For this review, take the finished solid that the model builds, in its own axes (mm). Coordinates: 2 decimals unless noted, no trailing zeros. Order: outer loops, then holes, each group sorted by start corner. A loop starts at its lowest first (then second) coordinate and runs counter-clockwise, first axis right, second up. Notation, with made-up numbers: (-30.75, 9.25) -> (0.25, 9.25) arc R13 ccw to (0.25, 21.25) -> close; hole circle Ø5 at (-30.5, 4). An arc over 180 degrees is marked (long way). Return JSON: item names as keys, results as strings. Group by question number.
Item 1: Take a section at C-C (x = -7). Write out the cut boundary in (y, z) (3 decimals).
Item 2: Insertion check: pin 1 (1.5 mm diameter, centred on x = -26, y = 1, fed in from +Z). The pin has a flat end and moves straight along its axis. Give the tip position at first contact, or say it passes through.
Item 3: Take a section at D-D (z = 1). Write out the cut boundary in (x, y) (3 decimals), then the cut area to 3 significant figures.
Item 4: For line 1 along Z through (x, y) = (0, 0.7) (3 decimals); line 2 along X through (y, z) = (2.35, 15); line 3 along Z through (x, y) = (9, 1.65), list the stretches that pass through material, from the lowest coordinate up.
Item 5: Take a section at B-B (y = 2.6). Write out the cut boundary in (x, z) (3 decimals), then the cut area to 3 significant figures.
Item 6: Take a section at A-A (x = 0). Write out the cut boundary in (y, z) (3 decimals), then the cut area to 3 significant figures.
```python
from build123d import *

# Parameters (mm, degrees)
SKETCH1_W                = 25.4
SKETCH1_H                = 50.8
BOSS_EXTRUDE1_DEPTH      = 3.175
M5_CLEARANCE_HOLE1_D     = 5.5
M5_CLEARANCE_HOLE1_DEPTH = 12.7
M5_CLEARANCE_HOLE1_TIP   = 1.652366702
FILLET1_R                = 12.7
FILLET2_R                = 3.175


with BuildPart() as part:
    # Sketch1 → Boss-Extrude1 (new body)
    with BuildSketch(Plane(origin=(0, 0, 0), x_dir=(1, 0, 0), z_dir=(0, 1, 0))):
        Polygon((-12.7, 25.4), (-20.429044148, 30.6757697), (-43.552280389, -4.091606348), (-12.7, -25.4), align=None)
        Rectangle(SKETCH1_W, SKETCH1_H)
    extrude(amount=BOSS_EXTRUDE1_DEPTH)

    # M5 Clearance Hole1
    with Locations(Plane(origin=(0, 0, 0), x_dir=(-1, 0, 0), z_dir=(0, -1, 0))):
        with Locations((0, 15.875), (0, -15.875)):
            Hole(M5_CLEARANCE_HOLE1_D / 2, depth=M5_CLEARANCE_HOLE1_DEPTH)
            with Locations((0, 0, -(M5_CLEARANCE_HOLE1_DEPTH + M5_CLEARANCE_HOLE1_TIP / 2))):  # 118° drill point
                Cone(0, M5_CLEARANCE_HOLE1_D / 2, M5_CLEARANCE_HOLE1_TIP, mode=Mode.SUBTRACT)

    # Fillet1
    fillet1_edges = [part.edges().sort_by_distance(p)[0] for p in [
        (-12.7, 1.5875, -25.4),
        (-12.7, 1.5875, 25.4),
    ]]
    fillet(fillet1_edges, radius=FILLET1_R)

    # Fillet2
    fillet2_edges = [part.edges().sort_by_distance(p)[0] for p in [
        (12.7, 1.5875, -25.4),
        (12.7, 1.5875, 25.4),
    ]]
    fillet(fillet2_edges, radius=FILLET2_R)


solid = part.part
```
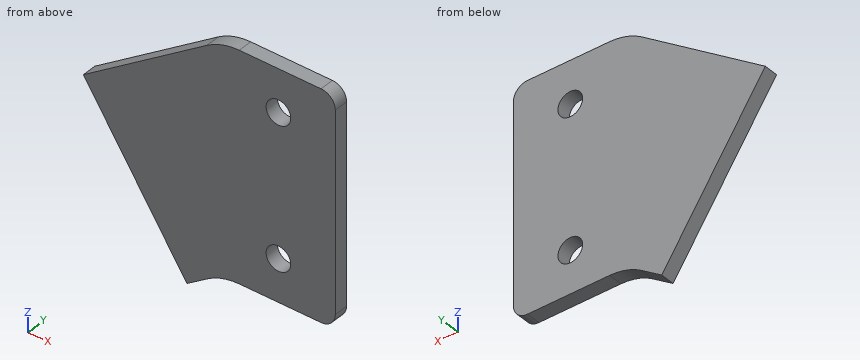
Findings below:
{
 "1": {"outline": "(0, -25.4) -> (3.175, -25.4) -> (3.175, 25.4) -> (0, 25.4) -> close"},
 "2": {"pin 1": "stops at z = 16.73"},
 "3": {"outline": "(-41.496, 0) -> (12.7, 0) -> (12.7, 3.175) -> (-41.496, 3.175) -> close", "area": "172 mm2"},
 "4": {"line 1": "z = -25.4 to -18.625, -13.125 to 13.125, 18.625 to 25.4", "line 2": "x = -27.76 to -2.61, 2.61 to 12.7", "line 3": "z = -25.4 to 25.4"},
 "5": {"outline": "(-43.552, 4.092) -> (-20.429, -30.676) -> (-15.939, -27.611) arc R12.7 cw to (-8.779, -25.4) -> (9.525, -25.4) arc R3.175 ccw to (12.7, -22.225) -> (12.7, 22.225) arc R3.175 ccw to (9.525, 25.4) -> (-8.741, 25.4) arc R12.7 ccw to (-15.958, 23.15) -> close; hole circle Ø5.5 at (0, -15.875); hole circle Ø5.5 at (0, 15.875)", "area": "2,220 mm2"},
 "6": {"outline": "(0, -25.4) -> (3.175, -25.4) -> (3.175, -18.625) -> (0, -18.625) -> close; (0, -13.125) -> (3.175, -13.125) -> (3.175, 13.125) -> (0, 13.125) -> close; (0, 18.625) -> (3.175, 18.625) -> (3.175, 25.4) -> (0, 25.4) -> close", "area": "126 mm2"}
}
